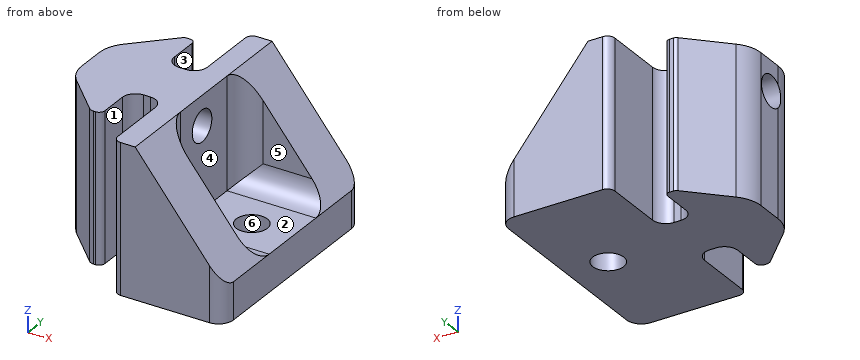
```python
from build123d import *

# Parameters (mm, degrees)
BOSS_EXTRUDE1_DEPTH = 20
CUT_EXTRUDE5_DEPTH  = 15
SKETCH3_R           = 2.1
CUT_EXTRUDE2_DEPTH  = 43.075221209
SKETCH5_R           = 2.1
CUT_EXTRUDE4_DEPTH  = 67.161318327
CUT_EXTRUDE6_DEPTH  = 65.034014837
FILLET1_R           = 3


with BuildPart() as part:
    # Sketch1 → Boss-Extrude1 (new body)
    with BuildSketch(Plane.XY):
        with BuildLine():
            Line((38.3, 10.745623604), (38.3, 9.881410941))
            Line((38.3, 9.881410941), (38.3, 5.394343623))
            ThreePointArc((38.3, 5.394343623), (38.592893219, 4.687236842), (39.3, 4.394343623))
            Line((39.3, 4.394343623), (40.3, 4.394343623))
            Line((40.3, 4.394343623), (51.3, 4.394343623))
            ThreePointArc((51.3, 4.394343623), (52.714213562, 4.98013006), (53.3, 6.394343623))
            Line((53.3, 6.394343623), (53.3, 29.710978016))
            Line((53.3, 29.710978016), (53.3, 31.710978016))
            ThreePointArc((53.3, 31.710978016), (52.714213562, 33.125191579), (51.3, 33.710978016))
            Line((51.3, 33.710978016), (41.3, 33.710978016))
            Line((41.3, 33.710978016), (39.3, 33.710978016))
            ThreePointArc((39.3, 33.710978016), (38.592893219, 33.418084798), (38.3, 32.710978016))
            Line((38.3, 32.710978016), (38.3, 28.215588568))
            Line((38.3, 28.215588568), (38.3, 27.353495632))
            Line((38.3, 27.353495632), (38.3, 24.630195866))
            ThreePointArc((38.3, 24.630195866), (37.780173169, 23.37522288), (36.525200183, 22.855396049))
            Line((36.525200183, 22.855396049), (35.6108, 22.855396049))
            ThreePointArc((35.6108, 22.855396049), (34.355826885, 23.375222934), (33.836, 24.630196049))
            Line((33.836, 24.630196049), (33.836, 28.448))
            ThreePointArc((33.836, 28.448), (33.634196572, 28.935196572), (33.147, 29.137))
            Line((33.147, 29.137), (32.664287242, 29.137))
            ThreePointArc((32.664287242, 29.137), (32.400617966, 29.084552836), (32.177090071, 28.935195973))
            Line((32.177090071, 28.935195973), (27.33900161, 24.097095612))
            ThreePointArc((27.33900161, 24.097095612), (26.352731832, 22.621035632), (26.0064, 20.879905136))
            Line((26.0064, 20.879905136), (26.0064, 17.220094864))
            ThreePointArc((26.0064, 17.220094864), (26.352731832, 15.478964368), (27.33900161, 14.002904388))
            Line((27.33900161, 14.002904388), (32.090366071, 9.25152824))
            ThreePointArc((32.090366071, 9.25152824), (32.409953896, 9.037986056), (32.786933649, 8.963))
            Line((32.786933649, 8.963), (33.060275787, 8.963))
            ThreePointArc((33.060275787, 8.963), (33.608795638, 9.190204362), (33.836, 9.738724213))
            Line((33.836, 9.738724213), (33.836, 13.469803585))
            ThreePointArc((33.836, 13.469803585), (34.355826992, 14.724776959), (35.610800366, 15.244603951))
            Line((35.610800366, 15.244603951), (36.5252, 15.244603951))
            ThreePointArc((36.5252, 15.244603951), (37.780173115, 14.724777066), (38.3, 13.469803951))
            Line((38.3, 13.469803951), (38.3, 10.745623604))
        make_face()
    extrude(amount=-BOSS_EXTRUDE1_DEPTH)

    # Sketch6 → Cut-Extrude5 (cut)
    with BuildSketch(Plane.XY):
        Polygon((53.3, 19.05266082), (53.3, 27.05266082), (41.3, 27.05266082), (41.3, 13.469803951), (41.3, 11.05266082), (53.3, 11.05266082), align=None)
    extrude(amount=-CUT_EXTRUDE5_DEPTH, mode=Mode.SUBTRACT)

    # Sketch3 → Cut-Extrude2 (cut, through all)
    with BuildSketch(Plane(origin=(41.3, 0, 0), x_dir=(0, 0, -1), z_dir=(1, 0, 0))):
        with Locations((4, 18.710978016)):
            Circle(SKETCH3_R)
    extrude(amount=-CUT_EXTRUDE2_DEPTH, mode=Mode.SUBTRACT)

    # Sketch5 → Cut-Extrude4 (cut, through all)
    with BuildSketch(Plane(origin=(0, 0, -20), x_dir=(-1, 0, 0), z_dir=(0, 0, -1))):
        with Locations((-47.8, 19.05266082)):
            Circle(SKETCH5_R)
    extrude(amount=-CUT_EXTRUDE4_DEPTH, mode=Mode.SUBTRACT)

    # Sketch7 → Cut-Extrude6 (cut, through all)
    with BuildSketch(Plane.XZ.offset(-4.394343623)):
        Polygon((41.3, 0), (53.3, -15), (53.3, 0), align=None)
    extrude(amount=-CUT_EXTRUDE6_DEPTH, mode=Mode.SUBTRACT)

    # Fillet1
    fillet1_edges = [part.edges().sort_by_distance(p)[0] for p in [
        (41.3, 11.05266082, -7.5),
        (41.3, 27.05266082, -7.5),
        (47.3, 11.05266082, -15),
        (47.3, 27.05266082, -15),
    ]]
    fillet(fillet1_edges, radius=FILLET1_R)


solid = part.part
```
Source: CAD feature listing. Evaluate the final solid. Frame: model axes, mm. Face numbers are marked on the shaded views. A direction names the side the tool comes from. Round coordinates to 2 decimals unless told otherwise and drop trailing zeros. Write each loop counter-clockwise with the first axis right and the second up, starting at its lowest first coordinate (ties: lowest second). Pieces come first, ordered by that corner, then holes. Notation, with made-up numbers: M 59,75 L 66,75 A10 cw 66,83 Z; hole C 55.25,56 d11. An arc over 180 degrees is marked long. Answer as a JSON object with one key per item and string values. Group by question number.
(1) Section query B-B on x = 48.25. Output: boundary loops of the cut face in (y, z).
(2) Mould query, pull axis X, two halves, no side actions, for the marked faces 4, 5 and 6. Classes: +X half, -X half, draft (parallel to the pull), parting line (faces both ways), or undercut.
(3) Ray query, line 1 (Y direction, x = 47.8, z = -16.2); line 2 (Z direction, x = 42.75, y = 22.25); line 3 (X direction, y = 28.25, z = -17.5). Return the intervals inside material, ascending. Write a range as [from, to].
(4) Reachability of the marked faces 1, 2 and 3 from +Z, -Z, +X, -X, +Y, -Y: full face, straight path, thin tool, end or side. Return the list, or none.
(5) Section query D-D on x = 43.5. Output: boundary loops of the cut face in (y, z), then the cut area to 3 significant figures.
(6) Section query C-C on y = 15.75. Output: boundary loops of the cut face in (x, z).
(7) First-contact query: pin 1 (5 mm diameter, centred on y = 17.5, z = -8, fed in from +X); pin 2 (4 mm diameter, centred on y = 16, z = -17, fed in from -X); pin 3 (8 mm diameter, centred on x = 30.5, z = -7.5, fed in from -Y); pin 4 (9 mm diameter, centred on y = 8.5, z = -10.5, fed in from -X). Flat tips, straight axial feed; report the tip coordinate or a pass-through.
Computed values:
{
 "1": {"outline": "M 4.39,-20 L 17,-20 L 17,-15 L 14.05,-15 A3 cw 11.05,-12 L 11.05,-8.69 L 4.39,-8.69 Z; M 21.1,-20 L 33.71,-20 L 33.71,-8.69 L 27.05,-8.69 L 27.05,-12 A3 cw 24.05,-15 L 21.1,-15 Z"},
 "2": {"face 4": "+X half", "face 5": "draft", "face 6": "undercut"},
 "3": {"line 1": "[4.39, 16.95], [21.15, 33.71]", "line 2": "[-20, -15]", "line 3": "[31.49, 33.84], [38.3, 53.3]"},
 "4": {"face 1": "+Z, -Z, -Y", "face 2": "+Z, +X", "face 3": "+Z, -Z, +Y"},
 "5": {"outline": "M 4.39,-20 L 33.71,-20 L 33.71,-2.75 L 26.94,-2.75 L 26.94,-12.8 A3 cw 24.05,-15 L 14.05,-15 A3 cw 11.16,-12.8 L 11.16,-2.75 L 4.39,-2.75 Z", "area": "316 mm^2"},
 "6": {"outline": "M 26.25,-20 L 53.3,-20 L 53.3,-15 L 41.3,-15 L 41.3,0 L 26.25,0 Z"},
 "7": {"pin 1": "x = 41.3", "pin 2": "x = 26.01", "pin 3": "y = 8.96", "pin 4": "x = 28.34"}
}
